from build123d import *

# Parameters (mm, degrees)
SZKIC1_W                    = 40
SZKIC1_H                    = 28
DODANIE_WYCI_GNI_CIE1_DEPTH = 2
ZAOKR_GLENIE1_SIZE          = 14
ZAOKR_GLENIE1_SIZE_2        = 8
SZKIC3_R                    = 1.6
SZKIC3_R_2                  = 5
WYTNIJ_WYCI_GNI_CIE1_DEPTH  = 29.653097735


with BuildPart() as part:
    # Szkic1 → Dodanie-wyciągnięcie1 (new body)
    with BuildSketch(Plane.XY):
        Rectangle(SZKIC1_W, SZKIC1_H)
    extrude(amount=DODANIE_WYCI_GNI_CIE1_DEPTH)

    # Zaokrąglenie1
    # an asymmetric fillet: 14, 8 mm, written as the material it takes off along each edge
    with BuildSketch(Plane(origin=(-20, 14, -35), x_dir=(1, 0, 0), z_dir=(0, 0, 1)), Plane(origin=(20, -14, -35), x_dir=(-1, 0, 0), z_dir=(0, 0, 1))) as zaokr_glenie1_piece_1:
        with BuildLine():
            Bezier((ZAOKR_GLENIE1_SIZE, 0), (0, 0), (0, -ZAOKR_GLENIE1_SIZE_2), weights=[1, 0.707106781, 1])
            Line((0, -ZAOKR_GLENIE1_SIZE_2), (0, 0))
            Line((0, 0), (ZAOKR_GLENIE1_SIZE, 0))
        make_face()
    extrude(amount=72, mode=Mode.SUBTRACT)
    with BuildSketch(Plane(origin=(-20, -14, -35), x_dir=(1, 0, 0), z_dir=(0, 0, 1))) as zaokr_glenie1_piece_2:
        with BuildLine():
            Bezier((ZAOKR_GLENIE1_SIZE, 0), (0, 0), (0, ZAOKR_GLENIE1_SIZE_2), weights=[1, 0.707106781, 1])
            Line((0, ZAOKR_GLENIE1_SIZE_2), (0, 0))
            Line((0, 0), (ZAOKR_GLENIE1_SIZE, 0))
        make_face()
    extrude(amount=72, mode=Mode.SUBTRACT)
    with BuildSketch(Plane(origin=(20, 14, -35), x_dir=(0, -1, 0), z_dir=(0, 0, 1))) as zaokr_glenie1_piece_3:
        with BuildLine():
            Bezier((ZAOKR_GLENIE1_SIZE_2, 0), (0, 0), (0, -ZAOKR_GLENIE1_SIZE), weights=[1, 0.707106781, 1])
            Line((0, -ZAOKR_GLENIE1_SIZE), (0, 0))
            Line((0, 0), (ZAOKR_GLENIE1_SIZE_2, 0))
        make_face()
    extrude(amount=72, mode=Mode.SUBTRACT)

    # Szkic3 → Wytnij-wyciągnięcie1 (cut, through all)
    with BuildSketch(Plane.XY.offset(15)):
        with Locations(Location((-15, -1e-09, 0), (0, 0, 180))):
            Circle(SZKIC3_R)
        with Locations(Location((15, -1e-09, 0), (0, 0, 180))):
            Circle(SZKIC3_R)
        with Locations(Location((0, 0, 0), (0, 0, 180))):
            Circle(SZKIC3_R_2)
    extrude(amount=-WYTNIJ_WYCI_GNI_CIE1_DEPTH, mode=Mode.SUBTRACT)


solid = part.part
Can you work these out from the model? Positions are in its coordinate system, mm. Round coordinates to 2 decimals unless told otherwise and drop trailing zeros. Loops run counter-clockwise (first coordinate to the right, second up) from the corner with the lowest first, then second, coordinate; pieces in that order, holes last. Notation, with made-up numbers: (42, 28.25) - (63, 28.25) arc R12 cw to (63, 50.25) - close; hole circle Ø3 at (39.25, -29.5). An arc over 180 degrees is marked (long way). Answer in a Markdown table with one row per item. Add a question column.
Q1. I want a section at B-B on x = 1.5. List the corners of the cut face in (y, z) for me.
Q2. For pin 1 Ø12 at (x, y) = (14.5, 10.5) entering from -Z; pin 2 Ø1 at (x, z) = (8, 1.5) entering from -Y, each with a flat end and sliding along its axis, tell me the tip position at first contact or that it passes through.
Q3. I want a section at C-C on z = 1.3. Count the separate pieces of the cut face and the enclosed holes in it, and give its area (3 significant figures).
Q4. I want a section at A-A on y = 0. List the corners of the cut face in (x, z) for me, and give its area (3 significant figures).
Q5. We'd pull the mould along Y, two halves only. Please class faces 1 (the flat face through (0, -14, 1)), 2 (the flat face through (20, 0, 1)), 3 (the cylindrical face through (16.6, -0.07, 1.01)), 4 (the flat face through (0, 14, 1)): pulls with the +Y half, pulls with the -Y half, needs draft (parallel to the pull), parting line crosses it, or undercut.
Q6. I need wall thicknesses on L1, parallel to Y at x = 0, z = 1; L2, parallel to Y at x = 1, z = 0.9; L3, parallel to X at y = -11, z = 1.2. Which ranges of each line are inside material? Lowest first, please.
A:
| question | item | result |
|---|---|---|
| 1 | outline | (-14, 0) - (-4.77, 0) - (-4.77, 2) - (-14, 2) - close; (4.77, 0) - (14, 0) - (14, 2) - (4.77, 2) - close |
| 2 | pin 1 | z = 0 |
| 2 | pin 2 | y = -13.95 |
| 3 | separate pieces | 1 |
| 3 | enclosed holes | 3 |
| 3 | area | 929 mm^2 |
| 4 | outline | (-20, 0) - (-16.6, 0) - (-16.6, 2) - (-20, 2) - close; (-13.4, 0) - (-5, 0) - (-5, 2) - (-13.4, 2) - close; (5, 0) - (13.4, 0) - (13.4, 2) - (5, 2) - close; (16.6, 0) - (20, 0) - (20, 2) - (16.6, 2) - close |
| 4 | area | 47.2 mm^2 |
| 5 | face 1 | pulls with the -Y half |
| 5 | face 2 | needs draft |
| 5 | face 3 | undercut |
| 5 | face 4 | pulls with the +Y half |
| 6 | L1 | -14 to -5, 5 to 14 |
| 6 | L2 | -14 to -4.9, 4.9 to 14 |
| 6 | L3 | -16.93 to 16.93 |
